Here's how the part is built. I have some questions about the finished solid (model axes, mm). Face numbers are marked on the shaded views. Coordinates: 2 decimals unless noted, no trailing zeros. Loops run counter-clockwise (first coordinate to the right, second up) from the corner with the lowest first, then second, coordinate; pieces in that order, holes last. Notation, with made-up numbers: M 86,41.5 L 130,41.5 A21 cw 130,61.5 Z; hole C 55,-28.75 d2. An arc over 180 degrees is marked long. Use CSV: the item, a comma, the result in double quotes. Start each with the question number.
Q1. Please list where these lines run through material, in increasing order: probe 1 along Z at (x, y) = (-5.25, 3.75); probe 2 along Z at (x, y) = (-5.75, 1.7); probe 3 along X at (y, z) = (1.25, -19.5). Write a range as [from, to].
Q2. If we section it at C-C (z = -29): Please give me the cut outline in (x, y).
Q3. If we section it at A-A (y = 1.3): State how many separate pieces and enclosed holes the cut face has, and give its area (3 significant figures).
Q4. For pin 1 Ø1.1 at (x, z) = (-3.9, -31.19) entering from -Y; pin 2 Ø0.6 at (x, z) = (-3.5, -35.5) entering from -Y; pin 3 Ø1.6 at (x, z) = (-3.9, -23.39) entering from +Y, each with a flat end and sliding along its axis, tell me the tip position at first contact or that it passes through.
Q5. If we section it at D-D (y = 4.8): Please give me the cut outline in (x, z), and give its area (3 significant figures).
Q6. If we mould it in two halves opening along Z, with no side actions, what happens to the marked faces 1 and 2? For each: +Z half, -Z half, draft (parallel to the pull), parting line (faces both ways), or undercut.
Autodesk Inventor part; units mm, degrees
ref_plane "YZ Plane" through (0, 0, 0) normal (1, 0, 0) x (0, 1, 0)
ref_plane "XZ Plane" through (0, 0, 0) normal (0, 1, 0) x (-1, 0, 0)
ref_plane "XY Plane" through (0, 0, 0) normal (0, 0, 1) x (1, 0, 0)
sketch "Sketch1" plane through (0, 0, 0) normal (0, 1, 0) x (-1, 0, 0)
  line L0 (0, 0) -> (7.7978, 0)
  line L1 (7.7978, 0) -> (7.7978, -46.7868)
  line L2 (7.7978, -46.7868) -> (0, -46.7868)
  line L3 (0, -46.7868) -> (0, 0)
  dimension "d0" = 7.7978
  dimension "d1" = 46.7868
extrude "Extrusion1" add sketch "Sketch1" along normal blind 3.236
sketch "Sketch2" plane through (0, 3.236, 0) normal (0, 1, 0) x (1, 0, 0)
  line L0 (0, 0) -> (-3.8989, 0) construction
  line L1 (-3.8989, 0) -> (-3.8989, 3.8989) construction
  line L2 (-3.8989, 3.8989) -> (0, 3.8989) construction
  line L3 (0, 3.8989) -> (0, 0) construction
  circle A0 centre (-3.8989, 3.8989) radius 2.4498
  dimension "d4" = 3.8989
  dimension "d5" = 3.8989
  dimension "d6" = 4.8997
extrude "Extrusion2" add sketch "Sketch2" along normal blind 1.9837
pattern_linear "Rectangular Pattern1" count 6 spacing 7.7978 along (0, 0, -1) of "Extrusion2"
shell "Shell1" thickness 1.4732 removed faces 1 at (-2.5993, 0, -15.5956)
sketch "Sketch3" plane through (-6.3246, 1.7628, -1.4732) normal (0, -1, 0) x (1, 0, 0)
  circle A0 centre (2.4257, -2.4257) radius 2.4498 construction
  circle A1 centre (2.4257, -10.2235) radius 2.4498 construction
  line L0 (2.4257, -2.4257) -> (2.4257, -10.2235) construction
  circle A2 centre (2.4257, -6.3246) radius 0.6198
  circle A3 centre (2.4257, -6.3246) radius 1.4491
  point P0 (6.3246, 1.4732)
  dimension "d13" = 1.2395
extrude "Extrusion3" add sketch "Sketch3" along normal up to surface (1.7628 mm away)
pattern_linear "Rectangular Pattern2" count 5 spacing 7.7978 along (0, 0, -1) of "Extrusion3"
properties part number "1x6 short black pegged" material "ABS Plastic"
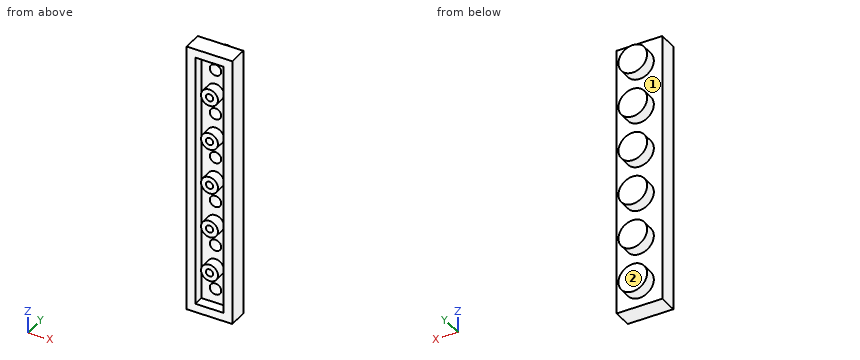
Results below:
1,probe 1,"[-44.93, -40.84], [-37.13, -33.05], [-29.34, -25.25], [-21.54, -17.45], [-13.74, -9.65], [-5.94, -1.86]"
1,probe 2,"[-46.79, -45.31], [-1.47, 0]"
1,probe 3,"[-7.8, -6.32], [-1.47, 0]"
2,outline,"M -7.8,0 L -6.32,0 L -6.32,1.76 L -1.47,1.76 L -1.47,0 L 0,0 L 0,3.24 L -2.14,3.24 L -2.14,5.22 L -5.66,5.22 L -5.66,3.24 L -7.8,3.24 Z"
3,separate pieces,"6"
3,enclosed holes,"6"
3,area,"179 mm^2"
4,pin 1,"y = 1.76"
4,pin 2,"y = 3.75"
4,pin 3,"y = 3.24"
5,outline,"C -3.9,-42.89 d4.9; C -3.9,-35.09 d4.9; C -3.9,-27.29 d4.9; C -3.9,-19.49 d4.9; C -3.9,-11.7 d4.9; C -3.9,-3.9 d4.9"
5,area,"113 mm^2"
6,face 1,"undercut"
6,face 2,"draft"
